Verification items for the finished model (mm, model axes). A direction names the side the tool comes from. Round coordinates to 2 decimals unless told otherwise and drop trailing zeros. Write each loop counter-clockwise with the first axis right and the second up, starting at its lowest first coordinate (ties: lowest second). Pieces come first, ordered by that corner, then holes. Notation, with made-up numbers: M 1.25,47 L 43.25,47 A23 ccw 43.25,56 Z; hole C 68,-25.5 d7. An arc over 180 degrees is marked long. One line per question, with ' | ' between items. Start each with the question number.
Q1. Cross-section at A-A (y = 9.5). Record the boundary of the cut face in (x, z).
Q2. Thickness scan on line 1 along Z through (x, y) = (1.25, 3); line 2 along Z through (x, y) = (0.9, 58.5); line 3 along X through (y, z) = (15.5, -5). Record the ranges inside material, lowest first. Write a range as from..to.
Q3. Tool access check on faces 4 (the face through (7.8, 24.1, -3.7)), 5 (the face through (8.39, 13.43, -2.85)). Record the directions out of +Z, -Z, +X, -X, +Y, -Y that give a thin tool (end or side, any length) a straight path to the whole face; none if there is none.
Q4. Cross-section at B-B (z = -4.5). State how many separate pieces and enclosed holes the cut face has, then the cut area to 3 significant figures.
Q5. Release check for a two-part mould opening along Y. For faces 1 (the face through (5.7, 26.1, -0.6)), 2 (the face through (1, 63, -4)), 3 (the face through (3, 31.1, -1.2)) record: released by +Y, released by -Y, zero draft, split by the parting line, or undercut.
Autodesk Inventor part; units mm, degrees
ref_plane "YZ Plane" through (0, 0, 0) normal (1, 0, 0) x (0, 1, 0)
ref_plane "XZ Plane" through (0, 0, 0) normal (0, 1, 0) x (-1, 0, 0)
ref_plane "XY Plane" through (0, 0, 0) normal (0, 0, 1) x (1, 0, 0)
sketch "スケッチ1" plane through (0, 0, 0) normal (0, 1, 0) x (-1, 0, 0)
  line L0 (0, 0) -> (-9, 0)
  line L1 (-9, 0) -> (-9, -9)
  line L2 (-9, -9) -> (0, -9)
  line L3 (0, -9) -> (0, 0)
  line L4 (-1.2, -1.2) -> (-7.8, -1.2)
  line L5 (-7.8, -1.2) -> (-7.8, -7.8)
  line L6 (-7.8, -7.8) -> (-1.2, -7.8)
  line L7 (-1.2, -7.8) -> (-1.2, -1.2)
  dimension "d0" = 9
  dimension "d1" = 9
  dimension "d2" = 1.2
  dimension "d3" = 1.2
  dimension "d4" = 1.2
  dimension "d5" = 1.2
extrude "押し出し1" add sketch "スケッチ1" along normal blind 63
sketch "スケッチ2" plane through (9, 0, 0) normal (1, 0, 0) x (0, 0, -1)
  line L0 (0, 63) -> (9, 63)
  line L1 (9, 0) -> (9, 63)
  line L2 (0, 0) -> (9, 0)
  point P0 (4.5, 58.5)
  point P1 (4.5, 13.5)
  dimension "d8" = 4.5
  dimension "d9" = 4.5
  dimension "d10" = 4.5
  dimension "d11" = 13.5
hole "穴1" at (9, 58.5, -4.5) at (9, 13.5, -4.5) direction (-1, 0, 0) diameter 3.3 end through all
sketch "スケッチ3" plane through (0, 0, 0) normal (0, 0, 1) x (1, 0, 0)
  line L0 (0, 0) -> (0, 63)
  line L1 (0, 0) -> (9, 0)
  line L2 (0, 63) -> (9, 63)
  point P0 (4.5, 49.5)
  point P1 (4.5, 4.5)
  dimension "d19" = 4.5
  dimension "d20" = 4.5
  dimension "d21" = 13.5
  dimension "d22" = 4.5
hole "穴2" at (4.5, 49.5, 0) at (4.5, 4.5, 0) direction (0, 0, -1) diameter 3.3 end through all
sketch "スケッチ4" plane through (9, 0, 0) normal (1, 0, 0) x (0, 0, -1)
  line L0 (0, 0) -> (9, 0)
  line L1 (9, 0) -> (9, 63)
  point P0 (4.5, 22)
  dimension "d30" = 22
  dimension "d31" = 4.5
hole "穴3" at (9, 22, -4.5) direction (-1, 0, 0) diameter 4 end through all
sketch "スケッチ5" plane through (0, 0, 0) normal (0, 0, 1) x (1, 0, 0)
  line L0 (0, 63) -> (9, 63)
  line L1 (9, 0) -> (9, 63)
  circle A0 centre (4.5, 49.5) radius 1.65
  point P0 (0, 0)
  point P1 (4.5, 56.25)
  point P2 (4.5, 44.5)
  point P3 (4.5, 39.5)
  point P4 (4.5, 34.5)
  point P5 (4.5, 29.5)
  point P6 (4.5, 24.5)
  point P7 (4.5, 19.5)
  point P8 (4.5, 14.5)
  point P9 (4.5, 9.5)
  dimension "d39" = 6.75
  dimension "d40" = 4.5
  dimension "d41" = 4.5
  dimension "d42" = 5
  dimension "d45" = 5
hole "穴4" at (4.5, 56.25, 0) at (4.5, 44.5, 0) at (4.5, 39.5, 0) at (4.5, 34.5, 0) at (4.5, 29.5, 0) at (4.5, 24.5, 0) at (4.5, 19.5, 0) at (4.5, 14.5, 0) at (4.5, 9.5, 0) direction (0, 0, -1) diameter 4 end through all
sketch "スケッチ7" plane through (9, 0, 0) normal (1, 0, 0) x (0, 0, -1)
  line L0 (0, 0) -> (0, 63)
  line L1 (0, 0) -> (9, 0)
  circle A0 centre (4.5, 22) radius 2
  point P0 (4.5, 6.75)
  point P1 (4.5, 27)
  point P2 (4.5, 32)
  point P3 (4.5, 37)
  point P4 (4.5, 42)
  point P5 (4.5, 47)
  point P6 (4.5, 52)
  dimension "d57" = 4.5
  dimension "d58" = 4.5
  dimension "d59" = 6.75
  dimension "d60" = 5
  dimension "d63" = 5
hole "穴5" at (9, 6.75, -4.5) at (9, 27, -4.5) at (9, 32, -4.5) at (9, 37, -4.5) at (9, 42, -4.5) at (9, 47, -4.5) at (9, 52, -4.5) direction (-1, 0, 0) diameter 4 end through all
equation "\"d4\" = d3"
equation "\"d5\" = d4"
properties part number "ハンド9x9_4" material "アルミニウム 6061"
Determined:
1) outline: M 0,-9 L 2.5,-9 L 2.5,-7.8 L 1.2,-7.8 L 1.2,-1.2 L 2.5,-1.2 L 2.5,0 L 0,0 Z; M 6.5,-9 L 9,-9 L 9,0 L 6.5,0 L 6.5,-1.2 L 7.8,-1.2 L 7.8,-7.8 L 6.5,-7.8 Z
2) line 1: z = -9..-7.8, -1.2..0 | line 2: z = -9..-6.15, -2.85..0 | line 3: x = 0..1.2, 7.8..9
3) face 4: +Y, -Y | face 5: +X, -X
4) separate pieces: 22 | enclosed holes: 0 | area: 58.6 mm²
5) face 1: undercut | face 2: released by +Y | face 3: zero draft
